Verification items for the finished model (mm, model axes). Round coordinates to 2 decimals unless told otherwise and drop trailing zeros. Write each loop counter-clockwise with the first axis right and the second up, starting at its lowest first coordinate (ties: lowest second). Pieces come first, ordered by that corner, then holes.
from build123d import *

# Parameters (mm, degrees)
SKETCH_1_R          = 2.5
SKETCH_1_R_2        = 2.3
EXTRUDE_1_DEPTH     = 6.3
SKETCH_2_R          = 2.5
EXTRUDE_2_DEPTH     = 1
SKETCH_4_R          = 0.425
CUT_EXTRUDE_1_DEPTH = 8.224264668
SKETCH_5_R          = 1.675
CUT_EXTRUDE_2_DEPTH = 0.6
SKETCH_6_R          = 2.2
CUT_EXTRUDE_3_DEPTH = 0.5
FILLET_1_R          = 0.1
FILLET_2_R          = 0.1
CHAMFER_2_SIZE      = 0.3
SKETCH_9_R          = 2.5
SKETCH_9_R_2        = 2.4
CUT_EXTRUDE_4_DEPTH = 0.2


with BuildPart() as part:
    # 스케치1 → 보스-돌출1 (new body)
    with BuildSketch(Plane.XY):
        Circle(SKETCH_1_R)
        Circle(SKETCH_1_R_2, mode=Mode.SUBTRACT)
    extrude(amount=EXTRUDE_1_DEPTH)

    # 스케치2 → 보스-돌출2 (add)
    with BuildSketch(Plane.XY.offset(6.3)):
        Circle(SKETCH_2_R)
    extrude(amount=EXTRUDE_2_DEPTH)

    # 스케치4 → 컷-돌출1 (cut, through all)
    with BuildSketch(Plane(origin=(0, 0, 6.3), x_dir=(-1, 0, 0), z_dir=(0, 0, -1))):
        Circle(SKETCH_4_R)
    extrude(amount=-CUT_EXTRUDE_1_DEPTH, mode=Mode.SUBTRACT)

    # 스케치5 → 컷-돌출2 (cut)
    with BuildSketch(Plane(origin=(0, 0, 6.3), x_dir=(-1, 0, 0), z_dir=(0, 0, -1))):
        Circle(SKETCH_5_R)
    extrude(amount=-CUT_EXTRUDE_2_DEPTH, mode=Mode.SUBTRACT)

    # 스케치6 → 컷-돌출3 (cut)
    with BuildSketch(Plane(origin=(0, 0, 6.3), x_dir=(-1, 0, 0), z_dir=(0, 0, -1))):
        Circle(SKETCH_6_R)
    extrude(amount=-CUT_EXTRUDE_3_DEPTH, mode=Mode.SUBTRACT)

    # 필렛1
    fillet_1_edges = [part.edges().sort_by_distance(p)[0] for p in [
        (2.2, 0, 6.3),
    ]]
    fillet(fillet_1_edges, radius=FILLET_1_R - 0.0001)  # a hair under: the kernel refuses the full size

    # 필렛2
    fillet_2_edges = [part.edges().sort_by_distance(p)[0] for p in [
        (1.675, 0, 6.8),
    ]]
    fillet(fillet_2_edges, radius=FILLET_2_R - 0.0001)  # a hair under: the kernel refuses the full size

    # 모따기2
    chamfer_2_edges = [part.edges().sort_by_distance(p)[0] for p in [
        (0.425, 0, 6.9),
    ]]
    chamfer(chamfer_2_edges, length=CHAMFER_2_SIZE)

    # 스케치9 → 컷-돌출4 (cut)
    with BuildSketch(Plane(origin=(0, 0, 0), x_dir=(-1, 0, 0), z_dir=(0, 0, -1))):
        Circle(SKETCH_9_R)
        Circle(SKETCH_9_R_2, mode=Mode.SUBTRACT)
    extrude(amount=-CUT_EXTRUDE_4_DEPTH, mode=Mode.SUBTRACT)


solid = part.part
Q1. Material ranges on line 1 along Y through (x, z) = (0, 6.6); line 2 along X through (y, z) = (0.05, 2.5), recorded low to high.
Recorded:
line 1: y = -2.5 to -2.2, 2.2 to 2.5
line 2: x = -2.5 to -2.3, 2.3 to 2.5
Q2. Depth check by flat-ended pin: P1, Ø1.3, axis at x = 0, y = 0, coming from the -Z side (3 decimals); P2, Ø1, axis at y = -1.5, z = 1, coming from the +X side; P3, Ø1, axis at y = -2, z = 2, coming from the -X side. Enter the tip coordinate at first touch or a pass-through.
Recorded:
P1: stops at z = 6.975
P2: stops at x = 2.29
P3: stops at x = -2
Q3. Sectioned sample at C-C (z = 5). Enter the section's corners in (x, y), plus the area to 3 significant figures.
Recorded:
outline: circle Ø5 at (0, 0); hole circle Ø4.6 at (0, 0)
area: 3.02 mm2
Q4. Release check for a two-part mould opening along Y. For faces 1 (the flat face through (1, 0, 7.3)), 2 (the cylindrical face through (-1.825, -1.4, 3.106)), 3 (the cylindrical face through (-0.54, -2.44, 3.7)), 4 (the flat face through (-1, 0, 6.9)) record: released by +Y, released by -Y, zero draft, split by the parting line, or undercut.
Recorded:
face 1: zero draft
face 2: undercut
face 3: split by the parting line
face 4: undercut
